Print and shaded views of the part. All mm, measured from the part's lowest x, y and z. A direction names the side the tool comes from. Coordinates: 2 decimals unless noted, no trailing zeros. Order: outer loops, then holes, each group sorted by start corner. A loop starts at its lowest first (then second) coordinate and runs counter-clockwise, first axis right, second up. Notation, with made-up numbers: M 69.5,39 L 124.5,39 A14 ccw 124.5,48 Z; hole C 44,37.25 d9. An arc over 180 degrees is marked long. Return JSON: item names as keys, results as strings.
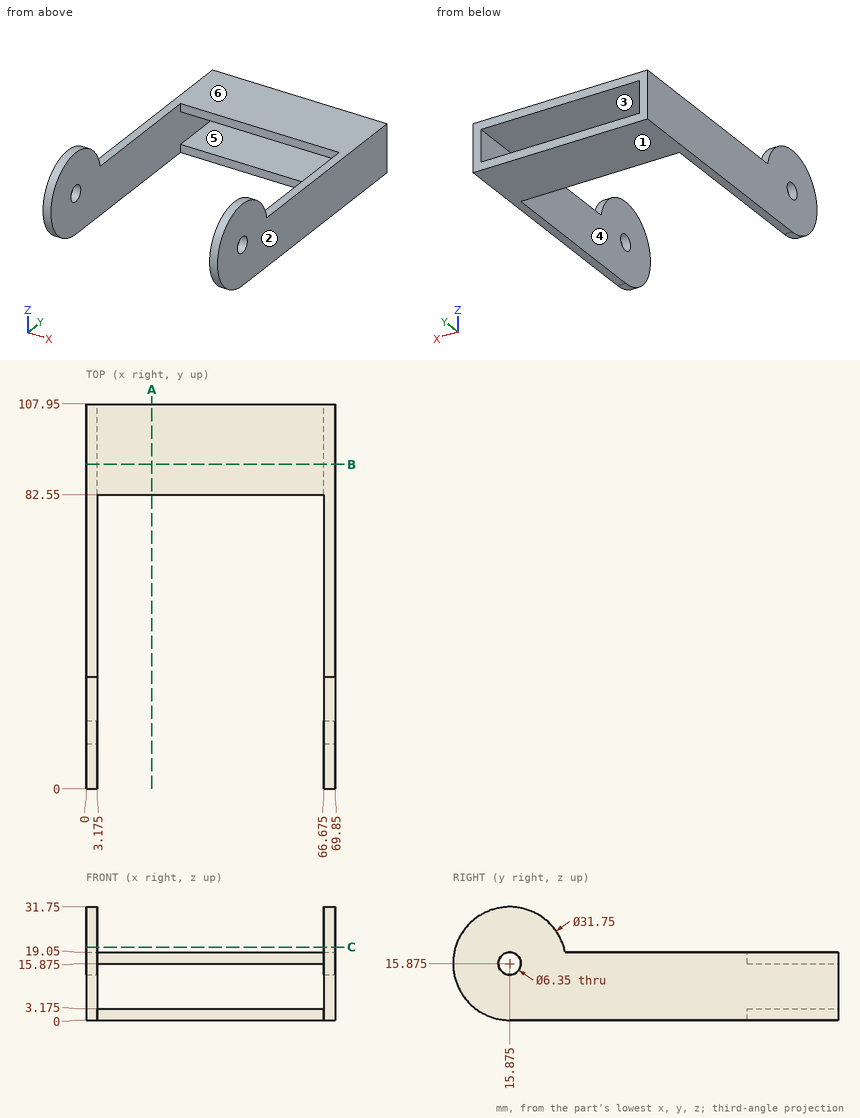
Item 1: Drop flat-ended pins along their axis: pin 1 Ø4 at (x, z) = (51, 6) entering from +Y; pin 2 Ø7.5 at (x, y) = (49.5, 97.5) entering from +Z; pin 3 Ø1.6 at (x, z) = (34.5, 1.5) entering from -Y. Give the stop position or say it passes through.
Check result:
{"pin 1": "passes through", "pin 2": "stops at z = 19.05", "pin 3": "stops at y = 82.55"}
Item 2: Pull direction Z, two halves, no side cores. Call the marked faces 1, 2 and 3: +Z half, -Z half, draft (parallel to the pull), parting line (faces both ways), or undercut.
Check result:
{"face 1": "-Z half", "face 2": "draft", "face 3": "undercut"}
Item 3: Wall check: line 1 (X direction, y = 95, z = 10) (3 decimals); line 2 (Z direction, x = 20, y = 93.5) (3 decimals); line 3 (Y direction, x = 54.5, z = 17). Give the ranges that are in metal, low to high.
Check result:
{"line 1": "x = 0 to 3.175, 66.675 to 69.85", "line 2": "z = 0 to 3.175, 15.875 to 19.05", "line 3": "y = 82.55 to 107.95"}
Item 4: 3-axis set-ups, long thin cutter, end or side, ignore diameter. For the marked faces 4, 5 and 6: which of +Z, -Z, +X, -X, +Y, -Y reach the whole face in a straight line?
Check result:
{"face 4": "-Y", "face 5": "+Y, -Y", "face 6": "+Z, +X, -X, +Y"}
Item 5: Saw through at A-A (x = 18.5). Write the cut outline in (y, z) (3 decimals).
Check result:
{"outline": "M 82.55,0 L 107.95,0 L 107.95,3.175 L 82.55,3.175 Z; M 82.55,15.875 L 107.95,15.875 L 107.95,19.05 L 82.55,19.05 Z"}
Item 6: Saw through at B-B (y = 91). Write the cut outline in (x, z) (3 decimals).
Check result:
{"outline": "M 0,0 L 69.85,0 L 69.85,19.05 L 0,19.05 Z; hole M 3.175,3.175 L 66.675,3.175 L 66.675,15.875 L 3.175,15.875 Z"}
Item 7: Saw through at C-C (z = 20.5). Write the cut outline in (x, y) (3 decimals).
Check result:
{"outline": "M 0,0.689 L 3.175,0.689 L 3.175,31.061 L 0,31.061 Z; M 66.675,0.689 L 69.85,0.689 L 69.85,31.061 L 66.675,31.061 Z"}
